```python
from build123d import *

# Parameters (mm, degrees)
SKETCH1_R           = 14.2875
SKETCH1_R_2         = 3.175
SKETCH1_W           = 38.1
SKETCH1_H           = 50.8
BOSS_EXTRUDE1_DEPTH = 3.175
FILLET1_R           = 3.81


with BuildPart() as part:
    # Sketch1 → Boss-Extrude1 (new body)
    with BuildSketch(Plane(origin=(0, 0, 0), x_dir=(1, 0, 0), z_dir=(0, 1, 0))):
        Polygon((0, 0), (0, 127), (152.4, 127), (203.2, 25.4), (203.2, 0), align=None)
        with Locations(Location((63.5, 101.6, 0), (0, 0, 270))):
            Circle(SKETCH1_R, mode=Mode.SUBTRACT)
        with Locations(Location((63.5, 66.04, 0), (0, 0, 270))):
            Circle(SKETCH1_R, mode=Mode.SUBTRACT)
        with Locations(Location((91.360222469, 43.942, 0), (0, 0, 270))):
            Circle(SKETCH1_R, mode=Mode.SUBTRACT)
        with Locations(Location((12.7, 12.7, 0), (0, 0, 270))):
            Circle(SKETCH1_R_2, mode=Mode.SUBTRACT)
        with Locations(Location((38.1, 12.7, 0), (0, 0, 270))):
            Circle(SKETCH1_R_2, mode=Mode.SUBTRACT)
        with Locations(Location((63.5, 12.7, 0), (0, 0, 270))):
            Circle(SKETCH1_R_2, mode=Mode.SUBTRACT)
        with Locations(Location((88.9, 12.7, 0), (0, 0, 270))):
            Circle(SKETCH1_R_2, mode=Mode.SUBTRACT)
        with Locations(Location((114.3, 12.7, 0), (0, 0, 270))):
            Circle(SKETCH1_R_2, mode=Mode.SUBTRACT)
        with Locations(Location((139.7, 12.7, 0), (0, 0, 270))):
            Circle(SKETCH1_R_2, mode=Mode.SUBTRACT)
        with Locations(Location((165.1, 12.7, 0), (0, 0, 270))):
            Circle(SKETCH1_R_2, mode=Mode.SUBTRACT)
        with Locations(Location((190.5, 12.7, 0), (0, 0, 270))):
            Circle(SKETCH1_R_2, mode=Mode.SUBTRACT)
        with Locations(Location((12.7, 38.1, 0), (0, 0, 270))):
            Circle(SKETCH1_R_2, mode=Mode.SUBTRACT)
        with Locations(Location((12.7, 63.5, 0), (0, 0, 270))):
            Circle(SKETCH1_R_2, mode=Mode.SUBTRACT)
        with Locations(Location((12.7, 88.9, 0), (0, 0, 270))):
            Circle(SKETCH1_R_2, mode=Mode.SUBTRACT)
        with Locations(Location((12.7, 114.3, 0), (0, 0, 270))):
            Circle(SKETCH1_R_2, mode=Mode.SUBTRACT)
        with Locations(Location((139.7, 38.1, 0), (0, 0, 270))):
            Circle(SKETCH1_R_2, mode=Mode.SUBTRACT)
        with Locations(Location((139.7, 63.5, 0), (0, 0, 270))):
            Circle(SKETCH1_R_2, mode=Mode.SUBTRACT)
        with Locations(Location((139.7, 88.9, 0), (0, 0, 270))):
            Circle(SKETCH1_R_2, mode=Mode.SUBTRACT)
        with Locations(Location((139.7, 114.3, 0), (0, 0, 270))):
            Circle(SKETCH1_R_2, mode=Mode.SUBTRACT)
        with Locations((107.95, 88.9)):
            Rectangle(SKETCH1_W, SKETCH1_H, mode=Mode.SUBTRACT)
    extrude(amount=BOSS_EXTRUDE1_DEPTH)

    # Fillet1
    fillet1_edges = [part.edges().sort_by_distance(p)[0] for p in [
        (88.9, 1.5875, -114.3),
        (88.9, 1.5875, -63.5),
        (127, 1.5875, -63.5),
        (127, 1.5875, -114.3),
        (0, 1.5875, 0),
        (0, 1.5875, -127),
        (152.4, 1.5875, -127),
        (203.2, 1.5875, -25.4),
        (203.2, 1.5875, 0),
    ]]
    fillet(fillet1_edges, radius=FILLET1_R)


solid = part.part
```
Verification items for the finished model (mm, model axes). Round coordinates to 2 decimals unless told otherwise and drop trailing zeros. Write each loop counter-clockwise with the first axis right and the second up, starting at its lowest first coordinate (ties: lowest second). Pieces come first, ordered by that corner, then holes. Notation, with made-up numbers: (10.5, -27.75) -> (45.5, -27.75) arc R15 cw to (45.5, -18.75) -> close; hole circle Ø4 at (18.5, 67). An arc over 180 degrees is marked (long way). Write each question's results on one line, items separated by ' | '. Start each with the question number.
1. Depth check by flat-ended pin: P1, Ø10, axis at x = 139.7, z = -38.1, coming from the +Y side (3 decimals); P2, Ø1, axis at y = 2, z = -97, coming from the +X side. Enter the tip coordinate at first touch or a pass-through.
2. Cross-section at A-A (x = 190.5). Enter the section's corners in (y, z) (3 decimals), then the cut area to 3 significant figures.
3. Cross-section at D-D (x = 165.1). Enter the section's corners in (y, z) (3 decimals), then the cut area to 3 significant figures.
4. Draft check along X on faces 1 (the cylindrical face through (162, 1.57, -13.39)), 2 (the flat face through (80, 0, -64)), 3 (the cylindrical face through (1.086, 1.61, -125.854)). Enter one of: +X half, -X half, draft (parallel to the pull), parting line (faces both ways), or undercut.
5. Cross-section at B-B (z = -103). Enter the section's corners in (x, y) (3 decimals), then the cut area to 3 significant figures.
6. Cross-section at C-C (x = 12.7). Enter the section's corners in (y, z) (3 decimals).
7. Material ranges on probe 1 along Z at (x, y) = (120.5, 0.2); probe 2 along X at (y, z) = (2.9, -95); probe 3 along Z at (x, y) = (57, 1.6), recorded low to high. Write a range as from..to.
Solutions:
1) P1: stops at y = 3.175 | P2: stops at x = 167.65
2) outline: (0, -50.8) -> (3.175, -50.8) -> (3.175, -15.875) -> (0, -15.875) -> close; (0, -9.525) -> (3.175, -9.525) -> (3.175, 0) -> (0, 0) -> close | area: 141 mm2
3) outline: (0, -101.6) -> (3.175, -101.6) -> (3.175, -15.875) -> (0, -15.875) -> close; (0, -9.525) -> (3.175, -9.525) -> (3.175, 0) -> (0, 0) -> close | area: 302 mm2
4) face 1: undercut | face 2: draft | face 3: -X half
5) outline: (0, 0) -> (49.281, 0) -> (49.281, 3.175) -> (0, 3.175) -> close; (77.719, 0) -> (88.9, 0) -> (88.9, 3.175) -> (77.719, 3.175) -> close; (127, 0) -> (164.4, 0) -> (164.4, 3.175) -> (127, 3.175) -> close | area: 311 mm2
6) outline: (0, -127) -> (3.175, -127) -> (3.175, -117.475) -> (0, -117.475) -> close; (0, -111.125) -> (3.175, -111.125) -> (3.175, -92.075) -> (0, -92.075) -> close; (0, -85.725) -> (3.175, -85.725) -> (3.175, -66.675) -> (0, -66.675) -> close; (0, -60.325) -> (3.175, -60.325) -> (3.175, -41.275) -> (0, -41.275) -> close; (0, -34.925) -> (3.175, -34.925) -> (3.175, -15.875) -> (0, -15.875) -> close; (0, -9.525) -> (3.175, -9.525) -> (3.175, 0) -> (0, 0) -> close
7) probe 1: z = -127..-114.3, -63.5..0 | probe 2: x = 0..50.83, 76.17..88.9, 127..168.4 | probe 3: z = -127..-114.32, -88.88..-78.76, -53.32..0
